Read the model definition and answer for the solid it produces. Units are mm, in the model's axes. Face numbers are marked on the shaded views. A direction names the side the tool comes from. Coordinates: 2 decimals unless noted, no trailing zeros. Write each loop counter-clockwise with the first axis right and the second up, starting at its lowest first coordinate (ties: lowest second). Pieces come first, ordered by that corner, then holes.
(1) Section B-B on y = -0.75 is taken. Write down the section's boundary in (x, z), then the cut area to 3 significant figures.
(2) The mould has two halves that part along Y. Classify the marked faces 1, 2 and 3: +Y half, -Y half, draft (parallel to the pull), parting line (faces both ways), or undercut.
(3) Find the intervals of material crossed by probe 1 along X at (y, z) = (0.5, 2.3); probe 2 along Y at (x, z) = (7.5, 2), in increasing order.
(4) Section A-A on z = 1.5 is taken. Write down the section's boundary in (x, y), then the cut area to 3 significant figures.
(5) Which of the six approach directions +Z, -Z, +X, -X, +Y, -Y give full straight-line access (tool end or side, diameter ignored) to the marked faces 4 and 5?
(6) Section C-C on x = 9.5 is taken. Write down the section's boundary in (y, z), then the cut area to 3 significant figures.
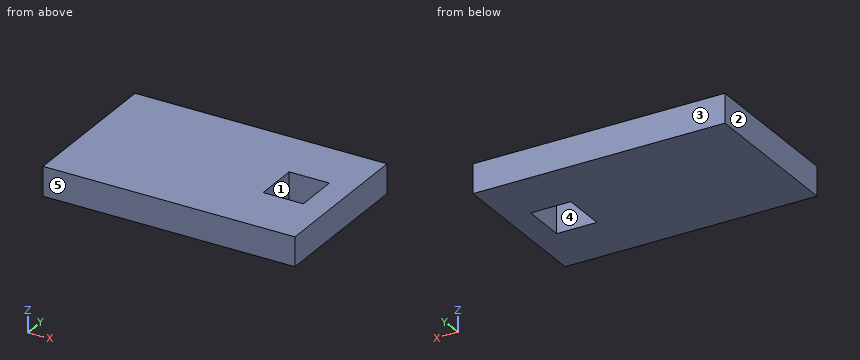
from build123d import *

# Parameters (mm, degrees)
IZIM1_W                     = 26
IZIM1_H                     = 16
IZIM1_R                     = 2.072340414
Y_KSEKLIK_EKSTR_ZYON1_DEPTH = 3
IZIM2_W                     = 4.147814154
IZIM2_H                     = 4.535167944
KES_EKSTR_ZYON1_DEPTH       = 10


with BuildPart() as part:
    # Çizim1 → Yükseklik-Ekstrüzyon1 (new body)
    with BuildSketch(Plane.XY):
        Rectangle(IZIM1_W, IZIM1_H)
        with Locations((8.385515416, 0)):
            Circle(IZIM1_R, mode=Mode.SUBTRACT)
    extrude(amount=Y_KSEKLIK_EKSTR_ZYON1_DEPTH)

    # Çizim2 → Kes-Ekstrüzyon1 (cut)
    with BuildSketch(Plane.XY.offset(3)):
        with Locations((8.385515416, 0)):
            Rectangle(IZIM2_W, IZIM2_H)
    extrude(amount=-KES_EKSTR_ZYON1_DEPTH, mode=Mode.SUBTRACT)


solid = part.part
Response:
1. outline: (-13, 0) - (6.31, 0) - (6.31, 3) - (-13, 3) - close; (10.46, 0) - (13, 0) - (13, 3) - (10.46, 3) - close
1. area: 65.6 mm2
2. face 1: undercut
2. face 2: draft
2. face 3: +Y half
3. probe 1: x = -13 to 6.31, 10.46 to 13
3. probe 2: y = -8 to -2.27, 2.27 to 8
4. outline: (-13, -8) - (13, -8) - (13, 8) - (-13, 8) - close; hole (6.31, -2.27) - (10.46, -2.27) - (10.46, 2.27) - (6.31, 2.27) - close
4. area: 397 mm2
5. face 4: +Z, -Z
5. face 5: +Z, -Z, +X, -X, -Y
6. outline: (-8, 0) - (-2.27, 0) - (-2.27, 3) - (-8, 3) - close; (2.27, 0) - (8, 0) - (8, 3) - (2.27, 3) - close
6. area: 34.4 mm2
